```python
from build123d import *

# Parameters (mm, degrees)
SKETCH1_W                                  = 180
SKETCH1_H                                  = 150
BOSS_EXTRUDE1_DEPTH                        = 15
SKETCH7_W                                  = 60
SKETCH7_H                                  = 25
BOSS_EXTRUDE6_DEPTH                        = 15
FILLET1_R                                  = 2
SKETCH2_W                                  = 38.5
SKETCH2_H                                  = 82
CUT_EXTRUDE1_DEPTH                         = 10
CUT_EXTRUDE3_DEPTH                         = 5
SKETCH11_W                                 = 5.5
SKETCH11_H                                 = 5.5
CUT_EXTRUDE6_DEPTH                         = 7
MIRROR3_AT_THE_SECOND_PLANE_COPY_1_SKETC_W = 5.5
MIRROR3_AT_THE_SECOND_PLANE_COPY_1_SKETC_H = 5.5
MIRROR3_AT_THE_SECOND_PLANE_COPY_1_DEPTH   = 7
MIRROR4_AT_THE_SECOND_PLANE_COPY_1_DEPTH   = 5
SKETCH12_W                                 = 194.678765725
SKETCH12_H                                 = 23.459831827
CUT_EXTRUDE7_DEPTH                         = 136.369863707


with BuildPart() as part:
    # Sketch1 → Boss-Extrude1 (new body)
    with BuildSketch(Plane(origin=(0, 0, 0), x_dir=(1, 0, 0), z_dir=(0, 1, 0))):
        Rectangle(SKETCH1_W, SKETCH1_H)
    extrude(amount=BOSS_EXTRUDE1_DEPTH)

    # Sketch7 → Boss-Extrude6 (add)
    with BuildSketch(Plane(origin=(0, 0, 0), x_dir=(1, 0, 0), z_dir=(0, 1, 0))):
        with Locations((0, -87.5)):
            Rectangle(SKETCH7_W, SKETCH7_H)
        with Locations((0, 87.5)):
            Rectangle(SKETCH7_W, SKETCH7_H)
    extrude(amount=BOSS_EXTRUDE6_DEPTH)

    # Fillet1
    fillet1_edges = [part.edges().sort_by_distance(p)[0] for p in [
        (-90, 15, 0),
        (60, 15, 75),
        (-60, 15, 75),
        (-30, 7.5, 100),
        (30, 7.5, 100),
        (-30, 15, 87.5),
        (0, 15, 100),
        (30, 15, 87.5),
        (-60, 15, -75),
        (0, 15, -100),
        (30, 7.5, -100),
        (-30, 15, -87.5),
        (-30, 7.5, -100),
        (30, 15, -87.5),
        (90, 15, 0),
        (90, 7.5, 75),
        (-90, 7.5, 75),
        (-90, 7.5, -75),
        (90, 7.5, -75),
        (60, 15, -75),
    ]]
    fillet(fillet1_edges, radius=FILLET1_R)

    # Sketch2 → Cut-Extrude1 (cut)
    with BuildSketch(Plane(origin=(0, 15, 0), x_dir=(1, 0, 0), z_dir=(0, 1, 0))):
        Rectangle(SKETCH2_W, SKETCH2_H)
    extrude(amount=-CUT_EXTRUDE1_DEPTH, mode=Mode.SUBTRACT)

    # Sketch10 → Cut-Extrude3 (cut)
    with BuildSketch(Plane(origin=(0, 15, 0), x_dir=(1, 0, 0), z_dir=(0, 1, 0))):
        Polygon((-9.25, -40.5), (-9.25, -33.162899401), (-4.25, -33.162899401), (-4.25, -40.5), (-4.25, -105.687952047), (-9.25, -105.687952047), align=None)
        Polygon((-99.022946063, 15), (-19.25, 15), (-11.555108838, 15), (-11.555108838, 10), (-19.25, 10), (-99.022946063, 10), align=None)
    cut_extrude3 = extrude(amount=-CUT_EXTRUDE3_DEPTH, mode=Mode.SUBTRACT)

    # Sketch11 → Cut-Extrude6 (cut)
    with BuildSketch(Plane(origin=(0, 15, 0), x_dir=(1, 0, 0), z_dir=(0, 1, 0))):
        with Locations((-21.549732367, 43.299732367)):
            Rectangle(SKETCH11_W, SKETCH11_H)
    cut_extrude6 = extrude(amount=-CUT_EXTRUDE6_DEPTH, mode=Mode.SUBTRACT)

    # Mirror3: Cut-Extrude6 across plane
    add(cut_extrude6.mirror(Plane(origin=(0, 0, 0), x_dir=(0, 0, 1), z_dir=(1, 0, 0))), mode=Mode.SUBTRACT)

    # Mirror3 at the second plane: Cut-Extrude6 across plane
    add(cut_extrude6.mirror(Plane.XY), mode=Mode.SUBTRACT)

    # Mirror3 at the second plane copy 1 sketc → Mirror3 at the second plane copy 1 (cut)
    with BuildSketch(Plane(origin=(0, 15, 0), x_dir=(-1, 0, 0), z_dir=(0, 1, 0))):
        with Locations((-21.549732367, 43.299732367)):
            Rectangle(MIRROR3_AT_THE_SECOND_PLANE_COPY_1_SKETC_W, MIRROR3_AT_THE_SECOND_PLANE_COPY_1_SKETC_H)
    extrude(amount=-MIRROR3_AT_THE_SECOND_PLANE_COPY_1_DEPTH, mode=Mode.SUBTRACT)

    # Mirror4: Cut-Extrude3 across plane
    add(cut_extrude3.mirror(Plane(origin=(0, 0, 0), x_dir=(0, 0, 1), z_dir=(1, 0, 0))), mode=Mode.SUBTRACT)

    # Mirror4 at the second plane: Cut-Extrude3 across plane
    add(cut_extrude3.mirror(Plane.XY), mode=Mode.SUBTRACT)

    # Mirror4 at the second plane copy 1 sketc → Mirror4 at the second plane copy 1 (cut)
    with BuildSketch(Plane(origin=(0, 15, 0), x_dir=(-1, 0, 0), z_dir=(0, 1, 0))):
        Polygon((-9.25, -40.5), (-9.25, -33.162899401), (-4.25, -33.162899401), (-4.25, -40.5), (-4.25, -105.687952047), (-9.25, -105.687952047), align=None)
        Polygon((-99.022946063, 15), (-19.25, 15), (-11.555108838, 15), (-11.555108838, 10), (-19.25, 10), (-99.022946063, 10), align=None)
    extrude(amount=-MIRROR4_AT_THE_SECOND_PLANE_COPY_1_DEPTH, mode=Mode.SUBTRACT)

    # Sketch12 → Cut-Extrude7 (cut, through all)
    with BuildSketch(Plane.XY):
        with Locations((1.797325826, 6.648635136)):
            Rectangle(SKETCH12_W, SKETCH12_H)
    extrude(amount=-CUT_EXTRUDE7_DEPTH, mode=Mode.SUBTRACT)


solid = part.part
```
Geometry check sheet. Reference: the model listing, model coordinates, mm. A direction names the side the tool comes from. Give positions to 0.01 mm unless a question says otherwise; leave off trailing zeros. Write each loop counter-clockwise with the first axis right and the second up, starting at its lowest first coordinate (ties: lowest second). Pieces come first, ordered by that corner, then holes. Notation, with made-up numbers: (-35, 71.5) -> (-21, 71.5) arc R20 ccw to (-21, 94.5) -> close; hole circle Ø10 at (-27.5, -9.75). An arc over 180 degrees is marked (long way). One line per question, with ' | ' between items.
Item 1: Depth check by flat-ended pin: pin 1 (6.5 mm diameter, centred on y = 5, z = 81.5, fed in from -X); pin 2 (3 mm diameter, centred on x = -65, y = 11.5, fed in from +Z). Enter the tip coordinate at first touch or a pass-through.
Determined:
pin 1: x = -30 | pin 2: z = 75
Item 2: Sectioned sample at D-D, the plane x = 13. Record the boundary of the cut face in (y, z).
Determined:
outline: (0, 0) -> (5, 0) -> (5, 41) -> (15, 41) -> (15, 98) arc R2 ccw to (13, 100) -> (0, 100) -> close
Item 3: Scan lines: line 1 along X through (y, z) = (8.5, 44); line 2 along X through (y, z) = (11.75, 80); line 3 along X through (y, z) = (12.5, 31). Record each from-to range of solid material in increasing order.
Determined:
line 1: -90 to -24.3, -18.8 to 18.8, 24.3 to 90 | line 2: -30 to -9.25, -4.25 to 4.25, 9.25 to 30 | line 3: -90 to -19.25, 19.25 to 90
Item 4: Sectioned sample at C-C, the plane z = 58.5. Record the boundary of the cut face in (x, y).
Determined:
outline: (-90, 0) -> (90, 0) -> (90, 13) arc R2 ccw to (88, 15) -> (9.25, 15) -> (9.25, 10) -> (4.25, 10) -> (4.25, 15) -> (-4.25, 15) -> (-4.25, 10) -> (-9.25, 10) -> (-9.25, 15) -> (-88, 15) arc R2 ccw to (-90, 13) -> close
Item 5: Sectioned sample at A-A, the plane z = 80.5. Record the boundary of the cut face in (x, y).
Determined:
outline: (-30, 0) -> (30, 0) -> (30, 13) arc R2 ccw to (28, 15) -> (9.25, 15) -> (9.25, 10) -> (4.25, 10) -> (4.25, 15) -> (-4.25, 15) -> (-4.25, 10) -> (-9.25, 10) -> (-9.25, 15) -> (-28, 15) arc R2 ccw to (-30, 13) -> close
Item 6: Access from +Z, -Z, +X, -X, +Y, -Y to the whole of each face (thin tool, end or side, straight path). Record for faces 1 (the flat face through (-30, 6, 87)), 2 (the flat face through (54, 13, 15)), 3 (the flat face through (-9.25, 13, 70)), 4 (the flat face through (24.3, 12, 43)), 5 (the flat face through (19.25, 10, 21)).
Determined:
face 1: +Z, -X, +Y, -Y | face 2: +X, -X, +Y | face 3: +Z, -Z, +Y | face 4: +Y | face 5: -Z, +Y
Item 7: Draft check along X on faces 6 (the flat face through (-90, 6, 37)), 7 (the flat face through (-1, 4, 0)), 8 (the flat face through (22, 12, 40.55)). Enter one of: released by +X, released by -X, zero draft, split by the parting line, or undercut.
Determined:
face 6: released by -X | face 7: zero draft | face 8: undercut
Item 8: Sectioned sample at B-B, the plane x = -60.5. Record the boundary of the cut face in (y, z).
Determined:
outline: (0, 0) -> (15, 0) -> (15, 10) -> (10, 10) -> (10, 15) -> (15, 15) -> (15, 73) arc R2 ccw to (13, 75) -> (0, 75) -> close
